Input: part model. Units: mm. Frame: model coordinates. A direction names the side the tool comes from. Give positions to 0.01 mm unless a question says otherwise; leave off trailing zeros. Write each loop counter-clockwise with the first axis right and the second up, starting at its lowest first coordinate (ties: lowest second). Pieces come first, ordered by that corner, then holes. Notation, with made-up numbers: (-11, -22.5) -> (7, -22.5) arc R16 cw to (7, -4.5) -> close; hole circle Ø6 at (-19.75, -12). An arc over 180 degrees is marked (long way). Answer as a JSON object with one key per item and string values. Group by question number.
from build123d import *

# Parameters (mm, degrees)
SKETCH_1_R          = 2
EXTRUDE_1_DEPTH     = 2
SKETCH_3_W          = 8.650610314
SKETCH_3_H          = 2
SKETCH_3_W_2        = 41.5
EXTRUDE_2_DEPTH     = 26
CUT_EXTRUDE_1_REACH = 51.47
SKETCH_4_R          = 2
CUT_EXTRUDE_2_REACH = 56.06
SKETCH_5_R          = 1.5
FILLET_1_R          = 3


with BuildPart() as part:
    # Sketch 1 → Extrude 1 (new body)
    with BuildSketch(Plane(origin=(0, 0, 0), x_dir=(1, 0, 0), z_dir=(0, 1, 0))):
        with BuildLine():
            Line((20.75, 0), (-20.75, 0))
            Line((-20.75, 0), (-20.75, 6.26619118))
            Line((-20.75, 6.26619118), (-25, 6.26619118))
            ThreePointArc((-25, 6.26619118), (-27.828427125, 7.437764055), (-29, 10.26619118))
            Line((-29, 10.26619118), (-29, 28.5))
            Line((-29, 28.5), (-20.349389686, 28.5))
            Line((-20.349389686, 28.5), (-20.349389686, 25.746501866))
            Line((-20.349389686, 25.746501866), (-19, 25.746501866))
            Line((-19, 25.746501866), (-19, 31.49))
            ThreePointArc((-19, 31.49), (-17.828427125, 34.318427125), (-15, 35.49))
            Line((-15, 35.49), (15, 35.49))
            ThreePointArc((15, 35.49), (17.828427125, 34.318427125), (19, 31.49))
            Line((19, 31.49), (19, 25.746501866))
            Line((19, 25.746501866), (20.349389686, 25.746501866))
            Line((20.349389686, 25.746501866), (20.349389686, 28.5))
            Line((20.349389686, 28.5), (29, 28.5))
            Line((29, 28.5), (29, 10.26619118))
            ThreePointArc((29, 10.26619118), (27.828427125, 7.437764055), (25, 6.26619118))
            Line((25, 6.26619118), (20.75, 6.26619118))
            Line((20.75, 6.26619118), (20.75, 0))
        make_face()
        with Locations(Location((-24.2, 22.5, 0), (0, 0, 270))):
            Circle(SKETCH_1_R, mode=Mode.SUBTRACT)
        with Locations(Location((-24.2, 12.5, 0), (0, 0, 270))):
            Circle(SKETCH_1_R, mode=Mode.SUBTRACT)
        with Locations(Location((24.2, 12.5, 0), (0, 0, 90))):
            Circle(SKETCH_1_R, mode=Mode.SUBTRACT)
        with Locations(Location((24.2, 22.5, 0), (0, 0, 90))):
            Circle(SKETCH_1_R, mode=Mode.SUBTRACT)
    extrude(amount=EXTRUDE_1_DEPTH)

    # Sketch 3 → Extrude 2 (add)
    with BuildSketch(Plane(origin=(0, 0, 0), x_dir=(1, 0, 0), z_dir=(0, 1, 0))):
        with Locations((-24.674694843, 29.5)):
            Rectangle(SKETCH_3_W, SKETCH_3_H)
        with Locations((24.674694843, 29.5)):
            Rectangle(SKETCH_3_W, SKETCH_3_H)
        with Locations((0, -1)):
            Rectangle(SKETCH_3_W_2, SKETCH_3_H)
    extrude(amount=EXTRUDE_2_DEPTH)

    # Sketch 4 → Cut-Extrude 1 (cut, up to next)
    with BuildSketch(Plane.XY.offset(-28.5), mode=Mode.PRIVATE) as cut_extrude_1_sk1:
        with Locations((-24.674694843, 19.5)):
            Circle(SKETCH_4_R)
    cut_extrude_1_tool1 = extrude(cut_extrude_1_sk1.sketch, amount=-CUT_EXTRUDE_1_REACH, mode=Mode.PRIVATE) & part.part
    # Sketch 4 → Cut-Extrude 1 (cut, up to next)
    with BuildSketch(Plane.XY.offset(-28.5), mode=Mode.PRIVATE) as cut_extrude_1_sk2:
        with Locations((-24.674694843, 7.6)):
            Circle(SKETCH_4_R)
    cut_extrude_1_tool2 = extrude(cut_extrude_1_sk2.sketch, amount=-CUT_EXTRUDE_1_REACH, mode=Mode.PRIVATE) & part.part
    cut_extrude_1_1 = cut_extrude_1_tool1.solids().sort_by_distance((-24.674695, 19.5, -28.5))[0]
    add(cut_extrude_1_1, mode=Mode.SUBTRACT)
    cut_extrude_1_2 = cut_extrude_1_tool2.solids().sort_by_distance((-24.674695, 7.6, -28.5))[0]
    add(cut_extrude_1_2, mode=Mode.SUBTRACT)
    cut_extrude_1 = cut_extrude_1_1 + cut_extrude_1_2  # Cut-Extrude 1 as one shape, for the pattern or mirror that repeats it

    # Sketch 5 → Cut-Extrude 2 (cut, up to next)
    with BuildSketch(Plane.XY.offset(2), mode=Mode.PRIVATE) as cut_extrude_2_sk1:
        with Locations((-10.25, 14.6)):
            Circle(SKETCH_5_R)
    cut_extrude_2_tool1 = extrude(cut_extrude_2_sk1.sketch, amount=-CUT_EXTRUDE_2_REACH, mode=Mode.PRIVATE) & part.part
    # Sketch 5 → Cut-Extrude 2 (cut, up to next)
    with BuildSketch(Plane.XY.offset(2), mode=Mode.PRIVATE) as cut_extrude_2_sk2:
        with Locations((-10.25, 21.6)):
            Circle(SKETCH_5_R)
    cut_extrude_2_tool2 = extrude(cut_extrude_2_sk2.sketch, amount=-CUT_EXTRUDE_2_REACH, mode=Mode.PRIVATE) & part.part
    # Sketch 5 → Cut-Extrude 2 (cut, up to next)
    with BuildSketch(Plane.XY.offset(2), mode=Mode.PRIVATE) as cut_extrude_2_sk3:
        with Locations((-3.25, 14.6)):
            Circle(SKETCH_5_R)
    cut_extrude_2_tool3 = extrude(cut_extrude_2_sk3.sketch, amount=-CUT_EXTRUDE_2_REACH, mode=Mode.PRIVATE) & part.part
    # Sketch 5 → Cut-Extrude 2 (cut, up to next)
    with BuildSketch(Plane.XY.offset(2), mode=Mode.PRIVATE) as cut_extrude_2_sk4:
        with Locations((-10.25, 7.6)):
            Circle(SKETCH_5_R)
    cut_extrude_2_tool4 = extrude(cut_extrude_2_sk4.sketch, amount=-CUT_EXTRUDE_2_REACH, mode=Mode.PRIVATE) & part.part
    # Sketch 5 → Cut-Extrude 2 (cut, up to next)
    with BuildSketch(Plane.XY.offset(2), mode=Mode.PRIVATE) as cut_extrude_2_sk5:
        with Locations((-17.25, 14.6)):
            Circle(SKETCH_5_R)
    cut_extrude_2_tool5 = extrude(cut_extrude_2_sk5.sketch, amount=-CUT_EXTRUDE_2_REACH, mode=Mode.PRIVATE) & part.part
    cut_extrude_2_1 = cut_extrude_2_tool1.solids().sort_by_distance((-10.25, 14.6, 2))[0]
    add(cut_extrude_2_1, mode=Mode.SUBTRACT)
    cut_extrude_2_2 = cut_extrude_2_tool2.solids().sort_by_distance((-10.25, 21.6, 2))[0]
    add(cut_extrude_2_2, mode=Mode.SUBTRACT)
    cut_extrude_2_3 = cut_extrude_2_tool3.solids().sort_by_distance((-3.25, 14.6, 2))[0]
    add(cut_extrude_2_3, mode=Mode.SUBTRACT)
    cut_extrude_2_4 = cut_extrude_2_tool4.solids().sort_by_distance((-10.25, 7.6, 2))[0]
    add(cut_extrude_2_4, mode=Mode.SUBTRACT)
    cut_extrude_2_5 = cut_extrude_2_tool5.solids().sort_by_distance((-17.25, 14.6, 2))[0]
    add(cut_extrude_2_5, mode=Mode.SUBTRACT)
    cut_extrude_2 = cut_extrude_2_1 + cut_extrude_2_2 + cut_extrude_2_3 + cut_extrude_2_4 + cut_extrude_2_5  # Cut-Extrude 2 as one shape, for the pattern or mirror that repeats it

    # Mirror 2: Cut-Extrude 1, Cut-Extrude 2 across plane
    add(cut_extrude_1.mirror(Plane.ZY), mode=Mode.SUBTRACT)
    add(cut_extrude_2.mirror(Plane.ZY), mode=Mode.SUBTRACT)

    # Fillet 1
    # the kernel refuses this fillet: 3 mm, written as the material it adds along each edge
    with BuildSketch(Plane(origin=(20.349389686, 2, -28.5), x_dir=(0, 0, 1), z_dir=(1, 0, 0)), Plane(origin=(-29, 2, -28.5), x_dir=(0, 0, 1), z_dir=(1, 0, 0))) as fillet_1_piece_1:
        with BuildLine():
            CenterArc((FILLET_1_R, -FILLET_1_R), FILLET_1_R, 90, 90)
            Line((0, -FILLET_1_R), (0, 0))
            Line((0, 0), (FILLET_1_R, 0))
        make_face()
    extrude(amount=8.650610314)
    with BuildSketch(Plane(origin=(20.75, 2, 0), x_dir=(0, 0, -1), z_dir=(-1, 0, 0))) as fillet_1_piece_2:
        with BuildLine():
            CenterArc((FILLET_1_R, -FILLET_1_R), FILLET_1_R, 90, 90)
            Line((0, -FILLET_1_R), (0, 0))
            Line((0, 0), (FILLET_1_R, 0))
        make_face()
    extrude(amount=41.5)
    # the kernel refuses this fillet: 3 mm, written as the material it takes off along each edge
    with BuildSketch(Plane(origin=(-12.849389686, 0, -30.5), x_dir=(0, 0, 1), z_dir=(-1, 0, 0))) as fillet_1_2_piece_1_section:
        with BuildLine():
            CenterArc((FILLET_1_R, FILLET_1_R), FILLET_1_R, 180, 90)
            Line((0, FILLET_1_R), (0, 0))
            Line((0, 0), (FILLET_1_R, 0))
        make_face()
    fillet_1_2_piece_1 = extrude(amount=23.650610314, mode=Mode.PRIVATE)
    fillet_1_2_piece_1 = split(fillet_1_2_piece_1, bisect_by=Plane(origin=(-19, 0.622520274, -29.811239081), z_dir=(-1, 0, 0)), keep=Keep.TOP, mode=Mode.PRIVATE)
    add(fillet_1_2_piece_1, mode=Mode.SUBTRACT)
    with BuildSketch(Plane(origin=(-29, 26, -38), x_dir=(0, -1, 0), z_dir=(0, 0, 1)), Plane(origin=(-20.349389686, 26, -21), x_dir=(0, -1, 0), z_dir=(0, 0, -1)), Plane(origin=(20.349389686, 26, -38), x_dir=(0, -1, 0), z_dir=(0, 0, 1)), Plane(origin=(29, 26, -21), x_dir=(0, -1, 0), z_dir=(0, 0, -1)), Plane(origin=(-20.75, 26, 9.5), x_dir=(1, 0, 0), z_dir=(0, 0, -1))) as fillet_1_2_piece_2:
        with BuildLine():
            CenterArc((FILLET_1_R, FILLET_1_R), FILLET_1_R, 180, 90)
            Line((0, FILLET_1_R), (0, 0))
            Line((0, 0), (FILLET_1_R, 0))
        make_face()
    extrude(amount=17, mode=Mode.SUBTRACT)
    with BuildSketch(Plane(origin=(36.5, 0, -30.5), x_dir=(0, 0, 1), z_dir=(-1, 0, 0))) as fillet_1_2_piece_3:
        with BuildLine():
            CenterArc((FILLET_1_R, FILLET_1_R), FILLET_1_R, 180, 90)
            Line((0, FILLET_1_R), (0, 0))
            Line((0, 0), (FILLET_1_R, 0))
        make_face()
    extrude(amount=16.150610314, mode=Mode.SUBTRACT)
    with BuildSketch(Plane(origin=(28.25, 0, 2), x_dir=(0, 0, -1), z_dir=(-1, 0, 0))) as fillet_1_2_piece_4:
        with BuildLine():
            CenterArc((FILLET_1_R, -FILLET_1_R), FILLET_1_R, 90, 90)
            Line((0, -FILLET_1_R), (0, 0))
            Line((0, 0), (FILLET_1_R, 0))
        make_face()
    extrude(amount=56.5, mode=Mode.SUBTRACT)
    with BuildSketch(Plane(origin=(20.75, 26, -7.5), x_dir=(0, -1, 0), z_dir=(0, 0, 1))) as fillet_1_2_piece_5:
        with BuildLine():
            CenterArc((FILLET_1_R, -FILLET_1_R), FILLET_1_R, 90, 90)
            Line((0, -FILLET_1_R), (0, 0))
            Line((0, 0), (FILLET_1_R, 0))
        make_face()
    extrude(amount=17, mode=Mode.SUBTRACT)


solid = part.part
1. Mould query, pull axis Y, two halves, no side actions, for faces 6 (the face through (0.29, 2.86, -0.9)), 7 (the face through (-11.36, 8.61, 1.01)), 8 (the face through (-22.217, 0.986, -12.76)). Classes: pulls with the +Y half, pulls with the -Y half, needs draft (parallel to the pull), parting line crosses it, or undercut.
2. Line query: line 1 (X direction, y = 0.8, z = -22.5); line 2 (Z direction, x = 24.2, y = 1.55); line 3 (Z direction, x = -12.5, y = 17.5). Output: solid intervals per line, ascending.
3. Section A-A (y = 7.6). Return the cut outline in (x, z), plus the area to 3 significant figures.
4. Section D-D (x = 10.25). Return the cut outline in (y, z).
5. Section C-C (z = -12.5). Return the cut outline in (x, y), plus the area to 3 significant figures.
6. Reachability of faces 1 (the face through (28.1, 25.14, -29.49)), 2 (the face through (-25, 14, -30.5)), 3 (the face through (23, 1, -6.266)), 4 (the face through (-20, 1, -25.747)), 5 (the face through (-20.75, 9, 1)) from +Z, -Z, +X, -X, +Y, -Y: full face, straight path, thin tool, end or side. Return the list, or none.
7. Contact query for flat-ended pins moving along their axis: pin 1 Ø2.5 at (x, y) = (23, 19.5) entering from -Z; pin 2 Ø5 at (y, z) = (4, -8) entering from -X; pin 3 Ø6 at (x, y) = (-11.5, 18.5) entering from -Z; pin 4 Ø2.5 at (x, y) = (10.25, 14.6) entering from -Z. Output: stop coordinate, or through.
8. Section B-B (x = 3.25). Return the cut outline in (y, z), plus the area to 3 significant figures.
Working result:
{
 "1": {"face 6": "pulls with the +Y half", "face 7": "undercut", "face 8": "needs draft"},
 "2": {"line 1": "x = -29 to -26.2, -22.2 to 22.2, 26.2 to 29", "line 2": "z = -30.13 to -24.5, -20.5 to -14.5, -10.5 to -6.27", "line 3": "z = 0 to 2"},
 "3": {"outline": "(-29, -30.5) -> (-26.67, -30.5) -> (-26.67, -28.5) -> (-29, -28.5) -> close; (-22.67, -30.5) -> (-20.35, -30.5) -> (-20.35, -28.5) -> (-22.67, -28.5) -> close; (-20.75, 0) -> (-11.75, 0) -> (-11.75, 2) -> (-20.75, 2) -> close; (-8.75, 0) -> (8.75, 0) -> (8.75, 2) -> (-8.75, 2) -> close; (11.75, 0) -> (20.75, 0) -> (20.75, 2) -> (11.75, 2) -> close; (20.35, -30.5) -> (22.67, -30.5) -> (22.67, -28.5) -> (20.35, -28.5) -> close; (26.67, -30.5) -> (29, -30.5) -> (29, -28.5) -> (26.67, -28.5) -> close", "area": "89.6 mm^2"},
 "4": {"outline": "(0, -35.49) -> (2, -35.49) -> (2, -3) arc R3 cw to (5, 0) -> (6.1, 0) -> (6.1, 2) -> (3, 2) arc R3 ccw to (0, -1) -> close; (9.1, 0) -> (13.1, 0) -> (13.1, 2) -> (9.1, 2) -> close; (16.1, 0) -> (20.1, 0) -> (20.1, 2) -> (16.1, 2) -> close; (23.1, 0) -> (26, 0) -> (26, 2) -> (23.1, 2) -> close"},
 "5": {"outline": "(-29, 0) -> (-26.2, 0) -> (-26.2, 2) -> (-29, 2) -> close; (-22.2, 0) -> (22.2, 0) -> (22.2, 2) -> (-22.2, 2) -> close; (26.2, 0) -> (29, 0) -> (29, 2) -> (26.2, 2) -> close", "area": "100 mm^2"},
 "6": {"face 1": "+Z, -Z, +X, +Y", "face 2": "-Z, +X, -X, +Y, -Y", "face 3": "+Z, +X, +Y, -Y", "face 4": "-Z, +Y, -Y", "face 5": "+Z, -X, +Y, -Y"},
 "7": {"pin 1": "stops at z = -30.5", "pin 2": "stops at x = -28.93", "pin 3": "stops at z = 0", "pin 4": "passes through"},
 "8": {"outline": "(0, -35.49) -> (2, -35.49) -> (2, -3) arc R3 cw to (5, 0) -> (13.1, 0) -> (13.1, 2) -> (3, 2) arc R3 ccw to (0, -1) -> close; (16.1, 0) -> (26, 0) -> (26, 2) -> (16.1, 2) -> close", "area": "117 mm^2"}
}
